```python
from build123d import *

# Parameters (mm, degrees)
F2_R             = 35.25
F3_DEPTH         = 11
F4_R             = 25
F7_R             = 17.5
F8_DEPTH         = 14.001
F9_R             = 5
F10_DEPTH        = 67.001
F10_COPIES_COUNT = 3
F11_R            = 52
F11_R_2          = 17.5
F12_DEPTH        = 67.001
F13_W            = 268.7109410763
F13_H            = 256.3393563032
F13_R            = 5
F13_R_2          = 52
F14_DEPTH        = 40
F15_R            = 63
F15_R_2          = 52
F16_DEPTH        = 1


# Not quite as in the source:
# - a feature of the source that left no trace in its solid (it failed there, or was rolled back) is left out
# - a pattern or mirror of a feature is missing from the dataset's text; its kind, count and spacing are read off the source's solid


with BuildPart() as f1:
    # F0 (on Front) → F1 (revolve)
    with BuildSketch(Plane.XZ):
        Polygon((67, 28.15), (67, 35.25), (0, 35.25), (0, 0), (14, 0), (14, 28.15), align=None)
    revolve(axis=Axis((7, 0, 0), (-1, 0, 0)))

    # F2 (on face) → F3 (join)
    with BuildSketch(Plane(origin=(0, 0, 0), x_dir=(0, -1, 0), z_dir=(-1, 0, 0))):
        Polygon((49.6521231503, 86), (-49.6521231503, 86), (-99.3042463006, 0), (-49.6521231503, -86), (49.6521231503, -86), (99.3042463006, 0), align=None)
        Circle(F2_R, mode=Mode.SUBTRACT)
    extrude(amount=-F3_DEPTH)

    # F4
    f4_edges = [f1.edges().sort_by_distance(p)[0] for p in [
        (5.5, 49.652123, -86),
        (5.5, -49.652123, -86),
        (5.5, -99.304246, 0),
        (5.5, -49.652123, 86),
        (5.5, 99.304246, 0),
        (5.5, 49.652123, 86),
    ]]
    fillet(f4_edges, radius=F4_R)

    # F7 (on face) → F8 (cut, through all)
    with BuildSketch(Plane.YZ.offset(14)):
        Circle(F7_R)
    extrude(amount=-F8_DEPTH, mode=Mode.SUBTRACT)

    # F9 (on face) → F10 (cut, through all)
    with BuildSketch(Plane(origin=(0, 0, 0), x_dir=(0, -1, 0), z_dir=(-1, 0, 0))):
        with Locations((-64.9519052838, -37.5)):
            Circle(F9_R)
    f10 = extrude(amount=-F10_DEPTH, mode=Mode.SUBTRACT)

    # F10_copies: F10 ×3 about axis
    f10_copies_axis = Axis((0, 0, 0), (1, 0, 0))
    for i in range(1, F10_COPIES_COUNT):
        add(f10.rotate(f10_copies_axis, i * 360 / F10_COPIES_COUNT), mode=Mode.SUBTRACT)

    # F11 (on face) → F12 (cut, through all)
    with BuildSketch(Plane(origin=(0, 0, 0), x_dir=(0, -1, 0), z_dir=(-1, 0, 0))):
        Circle(F11_R)
        Circle(F11_R_2, mode=Mode.SUBTRACT)
    extrude(amount=-F12_DEPTH, mode=Mode.SUBTRACT)

    # F13 (on face) → F14 (cut)
    with BuildSketch(Plane.YZ.offset(11)):
        with Locations((8.389338851, -8.3738937974)):
            Rectangle(F13_W, F13_H)
        with BuildLine():
            Line((-35.2183664206, 86), (35.2183664206, 86))
            ThreePointArc((35.2183664206, 86), (47.7183664206, 82.6506350946), (56.8690015152, 73.5))
            Line((56.8690015152, 73.5), (92.0873679357, 12.5))
            ThreePointArc((92.0873679357, 12.5), (95.4367328411, 0), (92.0873679357, -12.5))
            Line((92.0873679357, -12.5), (56.8690015152, -73.5))
            ThreePointArc((56.8690015152, -73.5), (47.7183664206, -82.6506350946), (35.2183664206, -86))
            Line((35.2183664206, -86), (-35.2183664206, -86))
            ThreePointArc((-35.2183664206, -86), (-47.7183664206, -82.6506350946), (-56.8690015152, -73.5))
            Line((-56.8690015152, -73.5), (-92.0873679357, -12.5))
            ThreePointArc((-92.0873679357, -12.5), (-95.4367328411, 0), (-92.0873679357, 12.5))
            Line((-92.0873679357, 12.5), (-56.8690015152, 73.5))
            ThreePointArc((-56.8690015152, 73.5), (-47.7183664206, 82.6506350946), (-35.2183664206, 86))
        make_face(mode=Mode.SUBTRACT)
        with BuildLine():
            ThreePointArc((56.8690015152, 73.5), (47.7183664206, 82.6506350946), (35.2183664206, 86))
            Line((35.2183664206, 86), (-35.2183664206, 86))
            ThreePointArc((-35.2183664206, 86), (-47.7183664206, 82.6506350946), (-56.8690015152, 73.5))
            Line((-56.8690015152, 73.5), (-92.0873679357, 12.5))
            ThreePointArc((-92.0873679357, 12.5), (-95.4367328411, 0), (-92.0873679357, -12.5))
            Line((-92.0873679357, -12.5), (-56.8690015152, -73.5))
            ThreePointArc((-56.8690015152, -73.5), (-47.7183664206, -82.6506350946), (-35.2183664206, -86))
            Line((-35.2183664206, -86), (35.2183664206, -86))
            ThreePointArc((35.2183664206, -86), (47.7183664206, -82.6506350946), (56.8690015152, -73.5))
            Line((56.8690015152, -73.5), (92.0873679357, -12.5))
            ThreePointArc((92.0873679357, -12.5), (95.4367328411, 0), (92.0873679357, 12.5))
            Line((92.0873679357, 12.5), (56.8690015152, 73.5))
        make_face()
        with Locations((-64.9519052838, -37.5)):
            Circle(F13_R, mode=Mode.SUBTRACT)
        with Locations((64.9519052838, -37.5)):
            Circle(F13_R, mode=Mode.SUBTRACT)
        Circle(F13_R_2, mode=Mode.SUBTRACT)
        with Locations((0, 75)):
            Circle(F13_R, mode=Mode.SUBTRACT)
    extrude(amount=F14_DEPTH, mode=Mode.SUBTRACT)

    # F15 (on face) → F16 (cut)
    with BuildSketch(Plane(origin=(0, 0, 0), x_dir=(0, -1, 0), z_dir=(-1, 0, 0))):
        Circle(F15_R)
        Circle(F15_R_2, mode=Mode.SUBTRACT)
    extrude(amount=-F16_DEPTH, mode=Mode.SUBTRACT)


solid = f1.part
```
CAD build for the part. Positions are in the model's coordinates, mm. Coordinates: 2 decimals unless noted, no trailing zeros. Write each loop counter-clockwise with the first axis right and the second up, starting at its lowest first coordinate (ties: lowest second). Pieces come first, ordered by that corner, then holes.
(1) Cut at B-B, the plane y = 0. List the corners of the cut face in (x, z), and give its area (3 significant figures).
(2) Two-plate mould, pull along Z, no slides. Class faces 1 (the face through (5.58, 47.56, 82.74)), 2 (the face through (11, 44, 39)), 3 (the face through (5.93, 41.265, -31.641)), 4 (the face through (5.577, -95.436, -0.183)): +Z half, -Z half, draft (parallel to the pull), parting line (faces both ways), or undercut.
(3) Cut at D-D, the plane z = -37.5. List the corners of the cut face in (x, y), and give its area (3 significant figures).
(4) Drill centre lines: probe 1 along Z at (x, y) = (0.45, 0); probe 2 along Z at (x, y) = (6.25, 0); probe 3 along X at (y, z) = (-54.5, -27). Where is each one in solid material? Low to high.
(5) Cut at A-A, the plane z = 0. List the corners of the cut face in (x, y), and give its area (3 significant figures).
(6) Flat gauge pins, fed straight in: pin 1 (8 mm diameter, centred on y = -38.5, z = -38.5, fed in from -X); pin 2 (1 mm diameter, centred on x = 9, y = -44.5, fed in from +Z). Where does each tip first touch, or does it go through?
(7) Cut at C-C, the plane y = 39.5. List the corners of the cut face in (x, z).
Geometry says:
1. outline: (0, -86) - (11, -86) - (11, -52) - (1, -52) - (1, -63) - (0, -63) - close; (0, 63) - (1, 63) - (1, 52) - (11, 52) - (11, 70) - (0, 70) - close; (0, 80) - (11, 80) - (11, 86) - (0, 86) - close
1. area: 616 mm2
2. face 1: +Z half
2. face 2: draft
2. face 3: undercut
2. face 4: parting line
3. outline: (0, -77.65) - (11, -77.65) - (11, -69.95) - (0, -69.95) - close; (0, -59.95) - (11, -59.95) - (11, -36.02) - (1, -36.02) - (1, -50.62) - (0, -50.62) - close; (0, 50.62) - (1, 50.62) - (1, 36.02) - (11, 36.02) - (11, 59.95) - (0, 59.95) - close; (0, 69.95) - (11, 69.95) - (11, 77.65) - (0, 77.65) - close
3. area: 667 mm2
4. probe 1: z = -86 to -63, 63 to 70, 80 to 86
4. probe 2: z = -86 to -52, 52 to 70, 80 to 86
4. probe 3: x = 1 to 11
5. outline: (0, -95.44) - (11, -95.44) - (11, -52) - (1, -52) - (1, -63) - (0, -63) - close; (0, 63) - (1, 63) - (1, 52) - (11, 52) - (11, 95.44) - (0, 95.44) - close
5. area: 934 mm2
6. pin 1: stops at x = 1
6. pin 2: stops at z = 84.41
7. outline: (0, -85.63) - (11, -85.63) - (11, -33.82) - (1, -33.82) - (1, -49.08) - (0, -49.08) - close; (0, 49.08) - (1, 49.08) - (1, 33.82) - (11, 33.82) - (11, 85.63) - (0, 85.63) - close
